from build123d import *

# Parameters (mm, degrees)
F0_W     = 5
F0_H     = 5
F1_DEPTH = 200
F3_DEPTH = 1.2
F5_DEPTH = 25
F6_D     = 3.3


with BuildPart() as f1:
    # F0 (on Right) → F1 (new body)
    with BuildSketch(Plane.YZ):
        Polygon((0, 30), (0, 15), (6.1031254008, 15), (10, 15), (10, 25), (15, 25), (20, 25), (20, 30), align=None)
        with Locations((17.5, 22.5)):
            Rectangle(F0_W, F0_H)
        with Locations((17.5, 7.5)):
            Rectangle(F0_W, F0_H)
        Polygon((0, 15), (0, 0), (20, 0), (20, 5), (15, 5), (10, 5), (10, 15), (6.1031254008, 15), align=None)
    extrude(amount=F1_DEPTH)

    # F2 (on face) → F3 (join)
    with BuildSketch(Plane.YZ.offset(200)):
        Polygon((20, 30), (0, 30), (0, 0), (20, 0), (20, 10), (15, 10), (15, 5), (10, 5), (10, 25), (15, 25), (15, 20), (20, 20), align=None)
        Polygon((20, 10), (20, 20), (15, 20), (15, 25), (10, 25), (10, 5), (15, 5), (15, 10), align=None)
    extrude(amount=F3_DEPTH)

    # F4 (on face) → F5 (cut)
    with BuildSketch(Plane(origin=(0, 10, 0), x_dir=(-1, 0, 0), z_dir=(0, 1, 0))):
        with BuildLine():
            ThreePointArc((-6.65, 15), (-5, 13.35), (-3.35, 15))
            Line((-3.35, 15), (-5, 15))
            Line((-5, 15), (-6.65, 15))
        make_face()
        with BuildLine():
            Line((-5, 15), (-3.35, 15))
            ThreePointArc((-3.35, 15), (-5, 16.65), (-6.65, 15))
            Line((-6.65, 15), (-5, 15))
        make_face()
    extrude(amount=-F5_DEPTH, mode=Mode.SUBTRACT)

    # F6 (through all)
    with Locations(Plane(origin=(0, 10, 0), x_dir=(-1, 0, 0), z_dir=(0, 1, 0))):
        with Locations((-15, 15), (-100, 15), (-185, 15)):
            Hole(F6_D / 2)


solid = f1.part
Can you work these out from the model? Positions are in its coordinate system, mm. A direction names the side the tool comes from. Give positions to 0.01 mm unless a question says otherwise; leave off trailing zeros. Loops run counter-clockwise (first coordinate to the right, second up) from the corner with the lowest first, then second, coordinate; pieces in that order, holes last. Notation, with made-up numbers: (-22, -22.5) - (3, -22.5) arc R14 ccw to (3, -13.5) - close; hole circle Ø3 at (-22, -4). An arc over 180 degrees is marked (long way). One line per item, written item: value.
(1) On a 3-axis mill with a long thin cutter (end or side, diameter ignored), from which of +Z, -Z, +X, -X, +Y, -Y can I reach the whole of each face in a straight line? I mean faces 4 (the face through (0, 8, 15)), 5 (the face through (99, 17, 20)), 6 (the face through (99, 15, 7)). Say none if no direction works.
Verdict:
face 4: +Z, -Z, -X, +Y, -Y
face 5: -X, +Y
face 6: -X
(2) If we section it at A-A, the plane x = 185: List the corners of the cut face in (y, z) for me, plus the area to 3 significant figures.
Verdict:
outline: (0, 0) - (20, 0) - (20, 10) - (15, 10) - (15, 5) - (10, 5) - (10, 13.35) - (0, 13.35) - close; (0, 16.65) - (10, 16.65) - (10, 25) - (15, 25) - (15, 20) - (20, 20) - (20, 30) - (0, 30) - close
area: 417 mm^2
(3) I'm going to push flat-ended pins straight in: pin 1 (12 mm diameter, centred on x = 36.5, z = 16.5, fed in from +Y); pin 2 (5.5 mm diameter, centred on x = 5, z = 15, fed in from +Y). Where does each tip first touch, or does it pass through?
Verdict:
pin 1: y = 20
pin 2: y = 10
(4) If we mould it in two halves opening along Y, with no side actions, what happens to faces 1 (the face through (99, 10, 13)), 2 (the face through (99, 0, 19)), 3 (the face through (99, 17, 10))? For each: released by +Y, released by -Y, zero draft, split by the parting line, or undercut.
Verdict:
face 1: undercut
face 2: released by -Y
face 3: zero draft
(5) I need wall thicknesses on line 1 along Z through (x, y) = (43, 16.5); line 2 along Z through (x, y) = (100, 6); line 3 along Y through (x, z) = (169, 21.5). Which ranges of each line are inside material? Lowest first, please.
Verdict:
line 1: 0 to 10, 20 to 30
line 2: 0 to 13.35, 16.65 to 30
line 3: 0 to 10, 15 to 20
